Here's how the part is built. I have some questions about the finished solid (model axes, mm). A direction names the side the tool comes from. Round coordinates to 2 decimals unless told otherwise and drop trailing zeros. Write each loop counter-clockwise with the first axis right and the second up, starting at its lowest first coordinate (ties: lowest second). Pieces come first, ordered by that corner, then holes. Notation, with made-up numbers: (48, 11) -> (77, 11) arc R25 cw to (77, 28) -> close; hole circle Ø1 at (17, 57). An arc over 180 degrees is marked (long way). Answer in a Markdown table with one row per item.
Autodesk Inventor part; units mm, degrees
ref_plane "Work Plane2" through (0, 0, 5) normal (0, 0, 1) x (1, 0, 0)
ref_plane "Work Plane8" through (0, 0, 0) normal (0.9510565, 0.309017, 0) x (0, 0, 1)
ref_plane "Work Plane9" through (0, 0, 0) normal (1, 0, 0) x (0, 1, 0)
sketch "Sketch1" plane through (0, 0, 0) normal (0, 0, 1) x (1, 0, 0)
  circle A0 centre (0, 0) radius 12
  dimension "d0" = 24
extrude "Extrusion1" add sketch "Sketch1" along normal blind 10
ref_plane "Work Plane2" through (0, 0, 5) normal (0, 0, 1) x (1, 0, 0)
sketch "Sketch2" plane through (0, 0, 0) normal (0, 0, -1) x (-1, 0, 0)
  circle A0 centre (0, 0) radius 12
  circle A1 centre (0, 0) radius 10
  dimension "d3" = 20
surface extrude "Pitch Diameter" sketch "Sketch2" against normal through all shown no curves A1
ref_plane "Work Plane8" through (0, 0, 0) normal (0.9510565, 0.309017, 0) x (0, 0, 1)
ref_plane "Work Plane9" through (0, 0, 0) normal (1, 0, 0) x (0, 1, 0)
spur gear teeth "Spur Gear" teeth 10 pitch diameter 20 tip diameter 24 root diameter 15 face width 10 start plane through (0, 0, 0) normal (0, 0, -1) x (-1, 0, 0)
equation "\"d0\" = da_da"
equation "\"d1\" = da_b"
equation "\"d3\" = da_d"
properties part number "Spur Gear1" material "Steel"
1) I want a section at A-A, the plane x = -10. List the corners of the cut face in (y, z) for me, and give its area (3 significant figures).
Response:
| item | result |
|---|---|
| outline | (-4.62, 0) -> (-1.63, 0) -> (-1.63, 10) -> (-4.62, 10) -> close; (1.63, 0) -> (4.62, 0) -> (4.62, 10) -> (1.63, 10) -> close |
| area | 59.7 mm^2 |
2) I need wall thicknesses on line 1 (Y direction, x = -9.5, z = 9); line 2 (Y direction, x = 8.5, z = 4); line 3 (Y direction, x = -6.5, z = 0.5). Which ranges of each line are inside material? Lowest first, please. Write a range as [from, to].
Response:
| item | result |
|---|---|
| line 1 | y = [-4.6, -1.37], [1.37, 4.6] |
| line 2 | y = [-4.48, -0.92], [0.92, 4.48] |
| line 3 | y = [-10.09, -6.01], [-3.96, 3.96], [6.01, 10.09] |
3) Which directions (+Z, -Z, +X, -X, +Y, -Y) give clear straight access to the entire face, cutting with the end or side of a thin tool? Please do faces 1 (the face through (6.996, 6.913, 4.93)), 2 (the face through (-4.413, 8.79, 4.93)), 3 (the face through (6.06, 4.42, 4.93)), 4 (the face through (-6.996, -6.913, 4.93)), 5 (the face through (-4.365, -8.743, 4.93)).
Response:
| item | result |
|---|---|
| face 1 | +Z, -Z, +X |
| face 2 | +Z, -Z, +Y |
| face 3 | +Z, -Z |
| face 4 | +Z, -Z, -X |
| face 5 | +Z, -Z, -Y |
4) I want a section at B-B, the plane y = 9.75. List the corners of the cut face in (x, z) for me.
Response:
| item | result |
|---|---|
| outline | (-7, 0) -> (-5.55, 0) -> (-5.55, 10) -> (-7, 10) -> close; (-1.59, 0) -> (1.59, 0) -> (1.59, 10) -> (-1.59, 10) -> close; (5.55, 0) -> (7, 0) -> (7, 10) -> (5.55, 10) -> close |
5) We'd pull the mould along X, two halves only. Please class faces 6 (the face through (-2.31, -7.135, 4.93)), 7 (the face through (11.41, 3.72, 4.93)), 8 (the face through (-11.41, -3.72, 4.93)), 9 (the face through (8.737, -4.517, 4.93)): +X half, -X half, draft (parallel to the pull), parting line (faces both ways), or undercut.
Response:
| item | result |
|---|---|
| face 6 | undercut |
| face 7 | +X half |
| face 8 | -X half |
| face 9 | undercut |
6) I want a section at D-D, the plane x = -4.5. List the corners of the cut face in (y, z) for me, and give its area (3 significant figures).
Response:
| item | result |
|---|---|
| outline | (-8.87, 0) -> (8.87, 0) -> (8.87, 10) -> (-8.87, 10) -> close |
| area | 177 mm^2 |
7) I want a section at C-C, the plane y = 0. List the corners of the cut face in (x, z) for me.
Response:
| item | result |
|---|---|
| outline | (-7.5, 0) -> (7.5, 0) -> (7.5, 10) -> (-7.5, 10) -> close |
8) For pin 1 (6 mm diameter, centred on y = -7, z = 5.5, fed in from +X); pin 2 (1.5 mm diameter, centred on x = 6, z = 5.5, fed in from -Y); pin 3 (4 mm diameter, centred on x = 9, z = 3, fed in from +Y), each with a flat end and sliding along its axis, tell me the tip position at first contact or that it passes through.
Response:
| item | result |
|---|---|
| pin 1 | stops at x = 11.31 |
| pin 2 | stops at y = -10.23 |
| pin 3 | stops at y = 9.75 |
